Geometry: final body of the model. Coordinates: model frame, mm. Face numbers are marked on the shaded views. A direction names the side the tool comes from. Round coordinates to 2 decimals unless told otherwise and drop trailing zeros. Write each loop counter-clockwise with the first axis right and the second up, starting at its lowest first coordinate (ties: lowest second). Pieces come first, ordered by that corner, then holes. Notation, with made-up numbers: (3.5, 50.25) - (45.5, 50.25) arc R27 cw to (45.5, 78.25) - close; hole circle Ø8 at (69, -8). An arc over 180 degrees is marked (long way). Use a Markdown table: item, result. Add a question column.
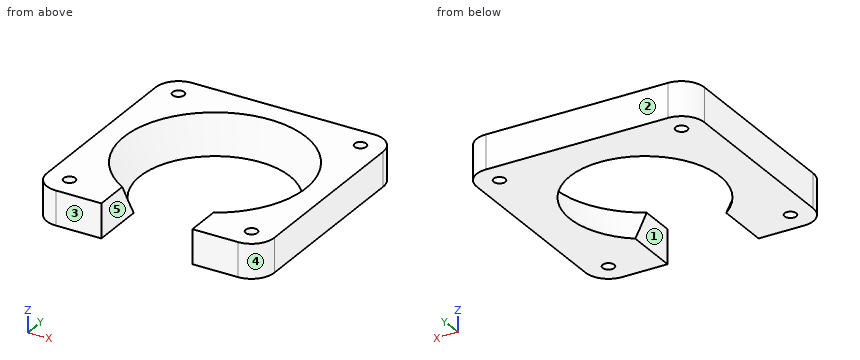
```python
from build123d import *

# Parameters (mm, degrees)
SKETCH1_W           = 63.5
SKETCH1_H           = 63.5
BOSS_EXTRUDE1_DEPTH = 9.525
SKETCH2_R           = 25.4
CUT_EXTRUDE1_DEPTH  = 12.7
CUT_EXTRUDE1_DRAFT  = -25
SKETCH3_W           = 25.4
SKETCH3_H           = 28.786668085
CUT_EXTRUDE2_DEPTH  = 9.525
SKETCH4_R           = 1.63195
CUT_EXTRUDE3_DEPTH  = 9.525
FILLET1_R           = 6.35
FILLET2_R           = 6.35


with BuildPart() as part:
    # Sketch1 → Boss-Extrude1 (new body)
    with BuildSketch(Plane.XY):
        with Locations((4.40013587, -6.298233696)):
            Rectangle(SKETCH1_W, SKETCH1_H)
    extrude(amount=BOSS_EXTRUDE1_DEPTH)


with BuildPart() as cut_extrude1_tool:
    # Sketch2 → Cut-Extrude1 (with draft: the straight prism first)
    with BuildSketch(Plane.XY.offset(9.525)):
        with Locations((4.40013587, -6.298233696)):
            Circle(SKETCH2_R)
    extrude(amount=-CUT_EXTRUDE1_DEPTH)
    # Cut-Extrude1: the draft: its side faces are tilted about the plane it starts from
    cut_extrude1_sides = [cut_extrude1_tool.faces().sort_by_distance(p)[0] for p in [
        (-20.99986413, -6.298233696, 3.175),
    ]]
    draft(cut_extrude1_sides, Plane.XY.offset(9.525), CUT_EXTRUDE1_DRAFT)


with BuildPart() as part_1:
    add(part.part)

    # Cut-Extrude1: cut by cut_extrude1_tool
    add(cut_extrude1_tool.part, mode=Mode.SUBTRACT)

    # Sketch3 → Cut-Extrude2 (cut)
    with BuildSketch(Plane.XY.offset(9.525)):
        with Locations((4.40013587, -23.654899654)):
            Rectangle(SKETCH3_W, SKETCH3_H)
    extrude(amount=-CUT_EXTRUDE2_DEPTH, mode=Mode.SUBTRACT)

    # Sketch4 → Cut-Extrude3 (cut)
    with BuildSketch(Plane.XY.offset(9.525)):
        with Locations((-20.99986413, 19.101766304)):
            Circle(SKETCH4_R)
        with Locations((29.80013587, 19.101766304)):
            Circle(SKETCH4_R)
        with Locations((29.80013587, -31.698233696)):
            Circle(SKETCH4_R)
        with Locations((-20.99986413, -31.698233696)):
            Circle(SKETCH4_R)
    extrude(amount=-CUT_EXTRUDE3_DEPTH, mode=Mode.SUBTRACT)

    # Fillet1
    fillet1_edges = [part_1.edges().sort_by_distance(p)[0] for p in [
        (-27.34986413, 25.451766304, 4.7625),
        (36.15013587, 25.451766304, 4.7625),
        (-27.34986413, -38.048233696, 4.7625),
    ]]
    fillet(fillet1_edges, radius=FILLET1_R)

    # Fillet2
    fillet2_edges = [part_1.edges().sort_by_distance(p)[0] for p in [
        (36.15013587, -38.048233696, 4.7625),
    ]]
    fillet(fillet2_edges, radius=FILLET2_R)


solid = part_1.part
```
1) Pin query (flat end, axial travel): P1, Ø4, axis at x = 5.5, z = 8, coming from the -Y side; P2, Ø3, axis at x = 9.5, z = 5.5, coming from the -Y side. Return the tip coordinate at first contact, or that it passes through.
2) Draft query along X for the marked faces 3, 4 and 5. Return one class per face: released by +X, released by -X, zero draft, split by the parting line, or undercut.
3) Section B-B, the plane z = 6.5. Return the cut outline in (x, y).
4) Material intervals for L1, parallel to X at y = -30, z = 2.75; L2, parallel to Y at x = 18.5, z = 6; L3, parallel to Y at x = 20.5, z = 3.25, sorted ascending. Write a range as from..to.
5) Set-up query: the marked faces 1 and 2. Return all of +Z, -Z, +X, -X, +Y, -Y with unobstructed straight access to the full face (end or side cutting, diameter ignored); none if empty.
6) Section A-A, the plane z = 2.5. Return the cut outline in (x, y).
Output values:
| question | item | result |
|---|---|---|
| 1 | P1 | stops at y = 17.43 |
| 1 | P2 | stops at y = 15.86 |
| 2 | face 3 | zero draft |
| 2 | face 4 | released by +X |
| 2 | face 5 | undercut |
| 3 | outline | (-27.35, -31.7) arc R6.35 ccw to (-21, -38.05) - (-8.3, -38.05) - (-8.3, -26.65) arc R23.99 cw (long way) to (17.1, -26.65) - (17.1, -38.05) - (29.8, -38.05) arc R6.35 ccw to (36.15, -31.7) - (36.15, 19.1) arc R6.35 ccw to (29.8, 25.45) - (-21, 25.45) arc R6.35 ccw to (-27.35, 19.1) - close; hole circle Ø3.26 at (-21, -31.7); hole circle Ø3.26 at (-21, 19.1); hole circle Ø3.26 at (29.8, -31.7); hole circle Ø3.26 at (29.8, 19.1) |
| 4 | L1 | x = -27.35..-8.3, 17.1..36.15 |
| 4 | L2 | y = -38.05..-25.42, 12.82..25.45 |
| 4 | L3 | y = -38.05..-21.98, 9.38..25.45 |
| 5 | face 1 | +Z, -Z, -Y |
| 5 | face 2 | +Z, -Z, +X, -X, +Y |
| 6 | outline | (-27.35, -31.7) arc R6.35 ccw to (-21, -38.05) - (-8.3, -38.05) - (-8.3, -24.41) arc R22.12 cw (long way) to (17.1, -24.41) - (17.1, -38.05) - (29.8, -38.05) arc R6.35 ccw to (36.15, -31.7) - (36.15, 19.1) arc R6.35 ccw to (29.8, 25.45) - (-21, 25.45) arc R6.35 ccw to (-27.35, 19.1) - close; hole circle Ø3.26 at (-21, -31.7); hole circle Ø3.26 at (-21, 19.1); hole circle Ø3.26 at (29.8, -31.7); hole circle Ø3.26 at (29.8, 19.1) |
